Work out the finished part from the listing and answer in its coordinate system (mm). Face numbers are marked on the shaded views. A direction names the side the tool comes from. Give positions to 0.01 mm unless a question says otherwise; leave off trailing zeros. Order: outer loops, then holes, each group sorted by start corner. A loop starts at its lowest first (then second) coordinate and runs counter-clockwise, first axis right, second up. Notation, with made-up numbers: (-7.5, 46.5) - (27.5, 46.5) arc R19 ccw to (27.5, 58.5) - close; hole circle Ø2 at (-25.5, 24.25). An arc over 180 degrees is marked (long way). Put each result on its own line as item: value.
```python
from build123d import *

# Parameters (mm, degrees)
SKETCH1_W           = 4.675
SKETCH1_H           = 0.825
BOSS_EXTRUDE1_DEPTH = 30


with BuildPart() as part:
    # Sketch1 → Boss-Extrude1 (new body)
    with BuildSketch(Plane.XY):
        with Locations((-3.3375, 1.6125)):
            Rectangle(SKETCH1_W, SKETCH1_H)
        with Locations((-3.3375, 0.4375)):
            Rectangle(SKETCH1_W, SKETCH1_H)
        Polygon((1, 2.025), (-1, 2.025), (-1, 1.2), (-0.475, 1.2), (-0.475, 0.85), (-1, 0.85), (-1, 0.025), (-1, -4), (-0.175, -4), (-0.175, 1.2), (0.175, 1.2), (0.175, -4), (1, -4), align=None)
    extrude(amount=BOSS_EXTRUDE1_DEPTH)


solid = part.part
```
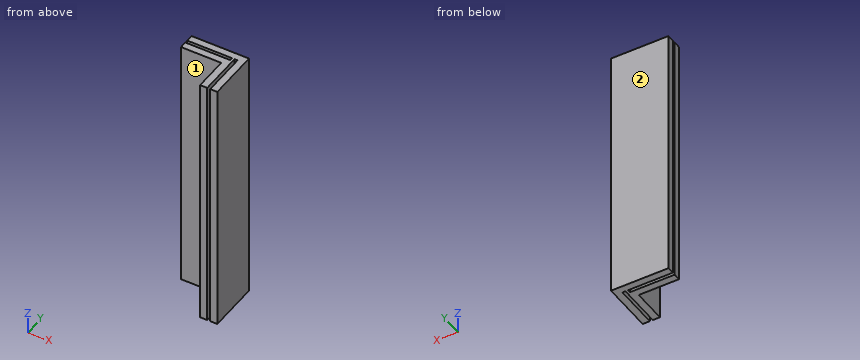
(1) Section C-C, the plane z = 19 is taken. Write down the section's boundary in (x, y) (3 decimals).
Geometry check:
outline: (-5.675, 0.025) - (-1, 0.025) - (-1, -4) - (-0.175, -4) - (-0.175, 1.2) - (0.175, 1.2) - (0.175, -4) - (1, -4) - (1, 2.025) - (-5.675, 2.025) - (-5.675, 1.2) - (-0.475, 1.2) - (-0.475, 0.85) - (-5.675, 0.85) - close
(2) Straight lines are drawn through the part: line 1 (Y direction, x = -3, z = 12) (3 decimals); line 2 (X direction, y = -3.25, z = 10) (3 decimals); line 3 (Y direction, x = -0.75, z = 4.5) (3 decimals). For each, find the intervals that lie inside material, in ascending order.
Geometry check:
line 1: y = 0.025 to 0.85, 1.2 to 2.025
line 2: x = -1 to -0.175, 0.175 to 1
line 3: y = -4 to 0.85, 1.2 to 2.025
(3) Section A-A, the plane x = -4.25 is taken. Write down the section's boundary in (y, z) (3 decimals), then the cut area to 3 significant figures.
Geometry check:
outline: (0.025, 0) - (0.85, 0) - (0.85, 30) - (0.025, 30) - close; (1.2, 0) - (2.025, 0) - (2.025, 30) - (1.2, 30) - close
area: 49.5 mm²
(4) Given pin 1 (1 mm diameter, centred on y = -1.5, z = 12, fed in from -X); pin 2 (1.4 mm diameter, centred on x = -3, z = 17, fed in from -Y) (3 decimals), each flat-ended and moving along its own axis, determine where each tip first touches the part or whether it passes through.
Geometry check:
pin 1: stops at x = -1
pin 2: stops at y = 0.025
(5) A tool of negligible diameter and unlimited length cuts with its end or side. For the marked faces 1 and 2, from which of +Z, -Z, +X, -X, +Y, -Y can it reach the whole face along a straight path? Write none if from no direction.
Geometry check:
face 1: +Z, -Z, -X, -Y
face 2: +Z, -Z, +X, -X, +Y
(6) Section B-B, the plane y = -1.75 is taken. Write down the section's boundary in (x, z) (3 decimals).
Geometry check:
outline: (-1, 0) - (-0.175, 0) - (-0.175, 30) - (-1, 30) - close; (0.175, 0) - (1, 0) - (1, 30) - (0.175, 30) - close
